from build123d import *

# Parameters (mm, degrees)
F_1_4_CLEARANCE_HOLE1_D = 6.7564
CIRPATTERN2_COUNT       = 10
F_3_8_CLEARANCE_HOLE1_D = 10.0838
SKETCH12_R              = 5.23875
CUT_EXTRUDE1_DEPTH      = 7.62


with BuildPart() as part:
    # Sketch1 → Revolve1 (revolve)
    with BuildSketch(Plane.XY):
        Polygon((0, -12.7), (-69.1515, -12.7), (-69.1515, 0), (-73.914, 0), (-73.914, -63.5), (-69.1515, -63.5), (-69.1515, -20.32), (0, -20.32), align=None)
    revolve(axis=Axis((0, 0, 0), (0, -1, 0)))

    # 1/4 Clearance Hole1 (through all)
    with Locations(Plane(origin=(0, -12.7, 0), x_dir=(1, 0, 0), z_dir=(0, 1, 0))):
        with Locations((0, 0)):
            Hole(F_1_4_CLEARANCE_HOLE1_D / 2)

    # Sketch7 → 1/8 (0.1250) Dowel Hole1 (revolve, cut)
    with BuildSketch(Plane(origin=(-73.914, -16.51, 0), x_dir=(0, 0, 1), z_dir=(0, 1, 0))):
        Polygon((0, 0), (0, 26.353866233), (1.5875, 25.4), (1.5875, 0), align=None)
    f_1_8_0_1250_dowel_hole1 = revolve(axis=Axis((-80.264, -16.51, 0), (1, 0, 0)), mode=Mode.SUBTRACT)

    # CirPattern2: 1/8 (0.1250) Dowel Hole1 ×10 about axis
    cirpattern2_axis = Axis((0, 0, 0), (0, 1, 0))
    for i in range(1, CIRPATTERN2_COUNT):
        add(f_1_8_0_1250_dowel_hole1.rotate(cirpattern2_axis, i * 360 / CIRPATTERN2_COUNT), mode=Mode.SUBTRACT)

    # 3/8 Clearance Hole1 (through all)
    with Locations(Plane(origin=(-26.9875, -12.7, 0), x_dir=(0, 0, 1), z_dir=(0, 1, 0))):
        with Locations((0, 0), (0, 53.975)):
            Hole(F_3_8_CLEARANCE_HOLE1_D / 2)

    # Sketch12 → Cut-Extrude1 (cut)
    with BuildSketch(Plane.XZ.offset(20.32)):
        with Locations((15.5575, 15.1384)):
            Circle(SKETCH12_R)
    extrude(amount=-CUT_EXTRUDE1_DEPTH, mode=Mode.SUBTRACT)


solid = part.part
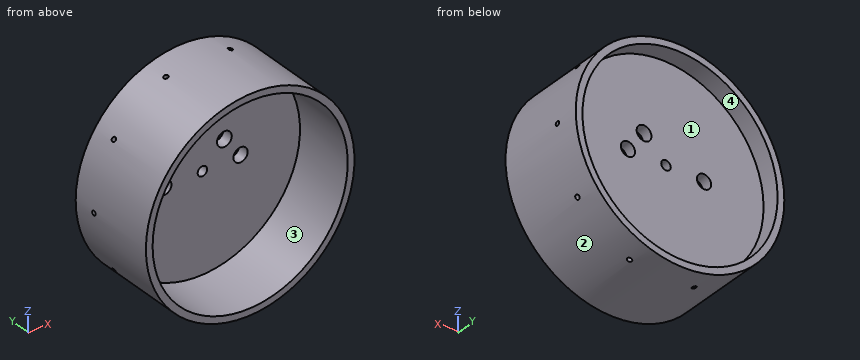
Input: part model. Units: mm. Frame: model coordinates. Face numbers are marked on the shaded views. A direction names the side the tool comes from. Coordinates: 2 decimals unless noted, no trailing zeros. Loops run counter-clockwise (first coordinate to the right, second up) from the corner with the lowest first, then second, coordinate; pieces in that order, holes last. Notation, with made-up numbers: (-27.75, 58.25) -> (-4.75, 58.25) arc R23 ccw to (-4.75, 82.25) -> close; hole circle Ø2 at (77.25, -1.5). An arc over 180 degrees is marked (long way). Write each question's results on one line, items separated by ' | '. Start each with the question number.
Q1. Section A-A, the plane x = 0. Return the cut outline in (y, z), plus the area to 3 significant figures.
Q2. Pull-direction query (X, two-part tool) for the marked faces 1 and 2; classes: released by +X, released by -X, zero draft, split by the parting line, or undercut.
Q3. Pin query (flat end, axial travel): pin 1 (1.9 mm diameter, centred on y = -16.51, z = 0, fed in from +X); pin 2 (2 mm diameter, centred on y = -38.5, z = -59, fed in from +X); pin 3 (9 mm diameter, centred on x = 0, z = 0, fed in from +Y). Return the tip coordinate at first contact, or that it passes through.
Q4. Section D-D, the plane z = 50.5. State how many separate pieces and enclosed holes the cut face has, plus the area to 3 significant figures.
Q5. Section C-C, the plane x = 35. Return the cut outline in (y, z), plus the area to 3 significant figures.
Q6. Ray query, line 1 (Y direction, x = -59.5, z = 0); line 2 (X direction, y = -48, z = -1.5); line 3 (Z direction, x = -2, y = -53). Return the intervals inside material, ascending. Write a range as from..to.
Q7. Reachability of the marked faces 3 and 4 from +Z, -Z, +X, -X, +Y, -Y: full face, straight path, thin tool, end or side. Return the list, or none.
Q8. Section B-B, the plane y = -56. Return the cut outline in (x, z).
Found:
1) outline: (-63.5, -73.91) -> (0, -73.91) -> (0, -69.15) -> (-12.7, -69.15) -> (-12.7, -3.38) -> (-20.32, -3.38) -> (-20.32, -69.15) -> (-63.5, -69.15) -> close; (-63.5, 69.15) -> (-20.32, 69.15) -> (-20.32, 3.38) -> (-12.7, 3.38) -> (-12.7, 69.15) -> (0, 69.15) -> (0, 73.91) -> (-63.5, 73.91) -> close | area: 1,610 mm2
2) face 1: undercut | face 2: split by the parting line
3) pin 1: x = 48.13 | pin 2: x = 45.82 | pin 3: y = -12.7
4) separate pieces: 1 | enclosed holes: 2 | area: 1,560 mm2
5) outline: (-63.5, -65.1) -> (0, -65.1) -> (0, -59.64) -> (-12.7, -59.64) -> (-12.7, 59.64) -> (0, 59.64) -> (0, 65.1) -> (-63.5, 65.1) -> (-63.5, 59.64) -> (-20.32, 59.64) -> (-20.32, -59.64) -> (-63.5, -59.64) -> close | area: 1,600 mm2
6) line 1: -20.32..-18.1, -14.92..-12.7 | line 2: -73.9..-69.14, 69.14..73.9 | line 3: -73.89..-69.12, 69.12..73.89
7) face 3: -Y | face 4: +Y
8) outline: circle Ø147.83 at (0, 0); hole circle Ø138.3 at (0, 0)
